```python
from build123d import *

# Parameters (mm, degrees)
BOSS_EXTRU_1_DEPTH      = 13.92
BOSS_EXTRU_2_DEPTH      = 1.5
ESQUISSE4_W             = 1.5
ESQUISSE4_H             = 0.855256697
ESQUISSE4_H_2           = 1.86
ESQUISSE4_H_3           = 3
ENL_V_MAT_EXTRU_1_DEPTH = 8
CHANFREIN1_SIZE         = 0.5


with BuildPart() as part:
    # Esquisse1 → Boss.-Extru.1 (new, symmetric)
    with BuildSketch(Plane(origin=(0, 0, 0), x_dir=(0, 1, 0), z_dir=(0, 0, 1))):
        Polygon((0, 3.879793809), (-3.36, 1.939896904), (-3.36, -1.939896904), (0, -3.879793809), (3.36, -1.939896904), (3.36, 1.939896904), align=None)
    extrude(amount=BOSS_EXTRU_1_DEPTH, both=True)

    # Esquisse2 → Boss.-Extru.2 (add)
    with BuildSketch(Plane.XY.offset(13.92)):
        Polygon((-1.939896904, 3.36), (-3.094597443, 3.36), (-5.034494347, 0), (-3.094597443, -3.36), (-1.939896904, -3.36), (-3.879793809, 0), align=None)
        Polygon((3.094597443, 3.36), (1.939896904, 3.36), (3.879793809, 0), (1.939896904, -3.36), (3.094597443, -3.36), (5.034494347, 0), align=None)
        Polygon((1.939896904, 3.36), (-1.939896904, 3.36), (-3.879793809, 0), (-1.939896904, -3.36), (1.939896904, -3.36), (3.879793809, 0), align=None)
    boss_extru_2 = extrude(amount=BOSS_EXTRU_2_DEPTH)

    # Esquisse4 → Enlèv. mat.-Extru.1 (cut)
    with BuildSketch(Plane.XY.offset(15.42)):
        with Locations((0, 3.787628349)):
            Rectangle(ESQUISSE4_W, ESQUISSE4_H)
        with Locations((0, 2.43)):
            Rectangle(ESQUISSE4_W, ESQUISSE4_H_2)
        Rectangle(ESQUISSE4_W, ESQUISSE4_H_3)
        with Locations((0, -2.43)):
            Rectangle(ESQUISSE4_W, ESQUISSE4_H_2)
        Polygon((0.75, 1.5), (0.75, -1.5), (0.866025404, -1.5), (1.732050808, 0), (0.866025404, 1.5), align=None)
        Polygon((-0.866025404, 1.5), (-1.732050808, 0), (-0.866025404, -1.5), (-0.75, -1.5), (-0.75, 1.5), align=None)
    enl_v_mat_extru_1 = extrude(amount=-ENL_V_MAT_EXTRU_1_DEPTH, mode=Mode.SUBTRACT)

    # Symétrie2: Boss.-Extru.2, Enlèv. mat.-Extru.1 across plane
    add(boss_extru_2.mirror(Plane.XY))
    add(enl_v_mat_extru_1.mirror(Plane.XY), mode=Mode.SUBTRACT)

    # Chanfrein1
    chanfrein1_edges = [part.edges().sort_by_distance(p)[0] for p in [
        (1.922298721, -3.36, -15.42),
        (1.922298721, 3.36, -15.42),
        (-1.922298721, 3.36, 15.42),
        (-1.922298721, -3.36, 15.42),
        (4.064545895, -1.68, 15.42),
        (4.064545895, 1.68, 15.42),
        (-4.064545895, 1.68, 15.42),
        (-4.064545895, -1.68, 15.42),
        (1.922298721, -3.36, 15.42),
        (1.922298721, 3.36, 15.42),
        (-4.064545895, -1.68, -15.42),
        (-4.064545895, 1.68, -15.42),
        (4.064545895, 1.68, -15.42),
        (4.064545895, -1.68, -15.42),
    ]]
    chamfer(chanfrein1_edges, length=CHANFREIN1_SIZE)


solid = part.part
```
Geometry check sheet. Reference: the model listing, model coordinates, mm. A direction names the side the tool comes from. Coordinates: 2 decimals unless noted, no trailing zeros. Order: outer loops, then holes, each group sorted by start corner. A loop starts at its lowest first (then second) coordinate and runs counter-clockwise, first axis right, second up.
Item 1: Depth check by flat-ended pin: pin 1 (1 mm diameter, centred on x = -1, y = 1, fed in from -Z); pin 2 (4 mm diameter, centred on y = 1, z = 3.5, fed in from -X); pin 3 (0.6 mm diameter, centred on y = -2.5, z = -11, fed in from +X); pin 4 (2 mm diameter, centred on y = 2.5, z = 11, fed in from +X). Enter the tip coordinate at first touch or a pass-through.
Item 2: Section check D-D (y = -0.5). Enter the section's corners in (x, z).
Item 3: Section check C-C (z = -3). Enter the section's corners in (x, y).
Item 4: Mould release check, pull along Y, two halves, no side actions. Record for faces 1 (the flat face through (-4.2, 0, -13.92)), 2 (the flat face through (-3.758, 1.704, -15.174)), 3 (the flat face through (-1.305, -0.74, 11.476)), 4 (the flat face through (-4.078, -1.656, -14.413)): released by +Y, released by -Y, zero draft, split by the parting line, or undercut.
Item 5: Section check B-B (x = 1.25). Enter the section's corners in (y, z).
Item 6: Tool access check on faces 5 (the flat face through (-2.9, -1.7, 0.2)), 6 (the flat face through (3.94, -0.23, -13.92)), 7 (the flat face through (2, 0, -15.42)), 8 (the flat face through (-1.293, 0.76, -11.476)), 9 (the flat face through (-3.837, 1.58, 15.167)). Record the directions out of +Z, -Z, +X, -X, +Y, -Y that give a thin tool (end or side, any length) a straight path to the whole face; none if there is none.
Item 7: Scan lines: line 1 along Z through (x, y) = (-3.5, -2.5); line 2 along X through (y, z) = (-1.75, -8.5); line 3 along X through (y, z) = (-2, 13). Record each from-to range of solid material in increasing order.
Item 8: Section check A-A (z = -8.5). Enter the section's corners in (x, y), plus the area to 3 significant figures.
Check sheet entries:
1. pin 1: stops at z = -15.42
1. pin 2: stops at x = -3.88
1. pin 3: stops at x = 2.61
1. pin 4: stops at x = 3.01
2. outline: (-4.75, -14.92) - (-4.17, -15.42) - (-1.44, -15.42) - (-1.44, -7.42) - (1.44, -7.42) - (1.44, -15.42) - (4.17, -15.42) - (4.75, -14.92) - (4.75, -13.92) - (3.59, -13.92) - (3.59, 13.92) - (4.75, 13.92) - (4.75, 14.92) - (4.17, 15.42) - (1.44, 15.42) - (1.44, 7.42) - (-1.44, 7.42) - (-1.44, 15.42) - (-4.17, 15.42) - (-4.75, 14.92) - (-4.75, 13.92) - (-3.59, 13.92) - (-3.59, -13.92) - (-4.75, -13.92) - close
3. outline: (-3.88, 0) - (-1.94, -3.36) - (1.94, -3.36) - (3.88, 0) - (1.94, 3.36) - (-1.94, 3.36) - close
4. face 1: zero draft
4. face 2: released by +Y
4. face 3: undercut
4. face 4: released by -Y
5. outline: (-3.36, -14.92) - (-2.86, -15.42) - (-0.83, -15.42) - (-0.83, -7.42) - (0.83, -7.42) - (0.83, -15.42) - (2.86, -15.42) - (3.36, -14.92) - (3.36, 14.92) - (2.86, 15.42) - (0.83, 15.42) - (0.83, 7.42) - (-0.83, 7.42) - (-0.83, 15.42) - (-2.86, 15.42) - (-3.36, 14.92) - close
6. face 5: -X, -Y
6. face 6: +X
6. face 7: -Z, +X, -X, +Y, -Y
6. face 8: -Z
6. face 9: +Z, -X, +Y
7. line 1: z = -15 to -13.92, 13.92 to 15
7. line 2: x = -2.87 to -0.75, 0.75 to 2.87
7. line 3: x = -2.73 to -0.75, 0.75 to 2.73
8. outline: (-3.88, 0) - (-1.94, -3.36) - (-0.75, -3.36) - (-0.75, -1.5) - (-0.87, -1.5) - (-1.73, 0) - (-0.87, 1.5) - (-0.75, 1.5) - (-0.75, 3.36) - (-1.94, 3.36) - close; (0.75, -3.36) - (1.94, -3.36) - (3.88, 0) - (1.94, 3.36) - (0.75, 3.36) - (0.75, 1.5) - (0.87, 1.5) - (1.73, 0) - (0.87, -1.5) - (0.75, -1.5) - close
8. area: 25.7 mm2
